```python
from build123d import *

# Parameters (mm, degrees)
F0_W      = 52.8
F0_H      = 20
F1_DEPTH  = 2.5
F2_W      = 40
F2_H      = 20
F3_DEPTH  = 6.85
F4_W      = 40
F4_H      = 20
F5_DEPTH  = 27
F6_R      = 2.2
F7_DEPTH  = 2.5
F8_W      = 0.7251760651
F8_H      = 2.6
F8_W_2    = 0.8560355749
F8_H_2    = 2.9239568868
F9_DEPTH  = 4
F10_W     = 0.7251760651
F10_H     = 2.6
F11_DEPTH = 5
F12_R     = 8
F13_DEPTH = 2.33
F14_R     = 2.5
F15_DEPTH = 4


with BuildPart() as f1:
    # F0 (on Top) → F1 (new body)
    with BuildSketch(Plane.XY):
        Rectangle(F0_W, F0_H)
    extrude(amount=F1_DEPTH)

    # F2 (on face) → F3 (join)
    with BuildSketch(Plane.XY.offset(2.5)):
        Rectangle(F2_W, F2_H)
    extrude(amount=F3_DEPTH)

    # F4 (on face) → F5 (join)
    with BuildSketch(Plane(origin=(0, 0, 0), x_dir=(1, 0, 0), z_dir=(0, 0, -1))):
        Rectangle(F4_W, F4_H)
    extrude(amount=F5_DEPTH)

    # F6 (on face) → F7 (cut, through all)
    with BuildSketch(Plane.XY.offset(2.5)):
        with Locations((-23.9, 5.1)):
            Circle(F6_R)
        with Locations((-23.9, -5.1)):
            Circle(F6_R)
        with Locations((23.9, 5.1)):
            Circle(F6_R)
        with Locations((23.9, -5.1)):
            Circle(F6_R)
    extrude(amount=-F7_DEPTH, mode=Mode.SUBTRACT)

    # F8 (on face) → F9 (cut)
    with BuildSketch(Plane.XY.offset(2.5)):
        with Locations((-26.0374119675, 5.1)):
            Rectangle(F8_W, F8_H)
        with Locations((-25.9719822126, -5.1)):
            Rectangle(F8_W_2, F8_H_2)
    extrude(amount=-F9_DEPTH, mode=Mode.SUBTRACT)

    # F10 (on face) → F11 (cut)
    with BuildSketch(Plane.XY.offset(2.5)):
        with Locations((26.0374119675, 5.1)):
            Rectangle(F10_W, F10_H)
        with Locations((26.0374119675, -5.1)):
            Rectangle(F10_W, F10_H)
    extrude(amount=-F11_DEPTH, mode=Mode.SUBTRACT)

    # F12 (on face) → F13 (join)
    with BuildSketch(Plane.XY.offset(9.35)):
        with Locations((-10.16, 0)):
            Circle(F12_R)
    extrude(amount=F13_DEPTH)

    # F14 (on face) → F15 (join)
    with BuildSketch(Plane.XY.offset(11.68)):
        with Locations((-10.16, 0)):
            Circle(F14_R)
    extrude(amount=F15_DEPTH)


solid = f1.part
```
The listing builds one solid part. Answer for the finished solid, in the listing's coordinates (mm). A direction names the side the tool comes from. Round coordinates to 2 decimals unless told otherwise and drop trailing zeros. Order: outer loops, then holes, each group sorted by start corner. A loop starts at its lowest first (then second) coordinate and runs counter-clockwise, first axis right, second up. Notation, with made-up numbers: (75.25, 25.5) -> (120.25, 25.5) arc R25 ccw to (120.25, 55.5) -> close; hole circle Ø11 at (-26.5, 19.5). An arc over 180 degrees is marked (long way). Answer as CSV lines item,"result".
Q1. Consider line 1 (Y direction, x = 23.9, z = 1.85); line 2 (Y direction, x = 23, z = 1); line 3 (X direction, y = -8, z = -5.5). Determine where each line is inside the solid, lowest interval first. Write a range as from..to.
Computed values:
line 1,"y = -10..-7.3, -2.9..2.9, 7.3..10"
line 2,"y = -10..-7.11, -3.09..3.09, 7.11..10"
line 3,"x = -20..20"
Q2. A cutting plane is placed at A-A on x = -23.9. Determine the outline of the cut face in (y, z).
Computed values:
outline,"(-10, 0) -> (-7.3, 0) -> (-7.3, 2.5) -> (-10, 2.5) -> close; (-2.9, 0) -> (2.9, 0) -> (2.9, 2.5) -> (-2.9, 2.5) -> close; (7.3, 0) -> (10, 0) -> (10, 2.5) -> (7.3, 2.5) -> close"
Q3. Given pin 1 (1 mm diameter, centred on x = 7, y = -5, fed in from +Z); pin 2 (5.5 mm diameter, centred on y = -1.5, z = 6.5, fed in from -X); pin 3 (5 mm diameter, centred on x = -23, y = 1.5, fed in from -Z); pin 4 (4 mm diameter, centred on x = -23.9, y = 5.1, fed in from -Z), each flat-ended and moving along its own axis, determine where each tip first touches the part or whether it passes through.
Computed values:
pin 1,"stops at z = 9.35"
pin 2,"stops at x = -20"
pin 3,"stops at z = 0"
pin 4,"passes through"
Q4. A cutting plane is placed at C-C on x = 7.5. Determine the outline of the cut face in (y, z).
Computed values:
outline,"(-10, -27) -> (10, -27) -> (10, 9.35) -> (-10, 9.35) -> close"
Q5. A cutting plane is placed at B-B on y = 0. Determine the outline of the cut face in (x, z).
Computed values:
outline,"(-26.4, 0) -> (-20, 0) -> (-20, -27) -> (20, -27) -> (20, 0) -> (26.4, 0) -> (26.4, 2.5) -> (20, 2.5) -> (20, 9.35) -> (-2.16, 9.35) -> (-2.16, 11.68) -> (-7.66, 11.68) -> (-7.66, 15.68) -> (-12.66, 15.68) -> (-12.66, 11.68) -> (-18.16, 11.68) -> (-18.16, 9.35) -> (-20, 9.35) -> (-20, 2.5) -> (-26.4, 2.5) -> close"
Q6. For a pull along X with two mould halves and no side action, classify faces 5 (the flat face through (-8, 2, 11.68)), 6 (the flat face through (-26.4, 8, 1)), 7 (the cylindrical face through (-21.7, 5.02, 1.27)) as +X half, -X half, draft (parallel to the pull), parting line (faces both ways), or undercut.
Computed values:
face 5,"draft"
face 6,"-X half"
face 7,"undercut"
Q7. A cutting plane is placed at D-D on z = -3.5. Determine the outline of the cut face in (x, y), plus the area to 3 significant figures.
Computed values:
outline,"(-20, -10) -> (20, -10) -> (20, 10) -> (-20, 10) -> close"
area,"800 mm^2"
Q8. Which of the six approach directions +Z, -Z, +X, -X, +Y, -Y give full straight-line access (tool end or side, diameter ignored) to faces 1 (the flat face through (23, 0, 2.5)), 2 (the flat face through (-20, 0, -13)), 3 (the flat face through (-23, 0, 2.5)), 4 (the flat face through (23, 0, 0))?
Computed values:
face 1,"+Z, +X, +Y, -Y"
face 2,"-Z, -X, +Y, -Y"
face 3,"+Z, -X, +Y, -Y"
face 4,"-Z, +X, +Y, -Y"
